Answer from the drawing. Dimensions are ordinates in mm from the lowest x, y and z of the part. A direction names the side the tool comes from. Coordinates: 2 decimals unless noted, no trailing zeros. Write each loop counter-clockwise with the first axis right and the second up, starting at its lowest first coordinate (ties: lowest second). Pieces come first, ordered by that corner, then holes. Notation, with made-up numbers: (-25, 49) - (0, 49) arc R29 cw to (0, 88) - close; hole circle Ø10 at (24.5, -8.5). An arc over 180 degrees is marked (long way). Use one line per item in the form item = value. Start each with the question number.
Item 1: A cutting plane is placed at B-B (z = 8.25). Write down the section's boundary in (x, y), then the cut area to 3 significant figures.
Item 2: Consider probe 1 along Y at (x, z) = (15, 2.75); probe 2 along Y at (x, z) = (18, 14.25); probe 3 along X at (y, z) = (169, 2). Determine where each line is inside the solid, lowest interval first.
Item 3: For the marked faces 1 and 2, determine the directions among +Z, -Z, +X, -X, +Y, -Y from which every point of the face is accessible in a straight line to the end or side of a thin tool.
Item 4: Given pin 1 (13 mm diameter, centred on x = 18, y = 19, fed in from +Z), flat-ended and moving along its own axis, determine where the tip first touches the part or whether it passes through.
Item 5: A cutting plane is placed at D-D (y = 19). Write down the section's boundary in (x, z), then the cut area to 3 significant figures.
Item 6: A cutting plane is placed at C-C (x = 18). Write down the section's boundary in (y, z), then the cut area to 3 significant figures.
Item 7: Determine the mould class of the marked faces 3, 4 and 5 for opening direction Y: released by +Y, released by -Y, zero draft, split by the parting line, or undercut.
Item 8: A cutting plane is placed at A-A (y = 163). Write down the section's boundary in (x, z), then the cut area to 3 significant figures.
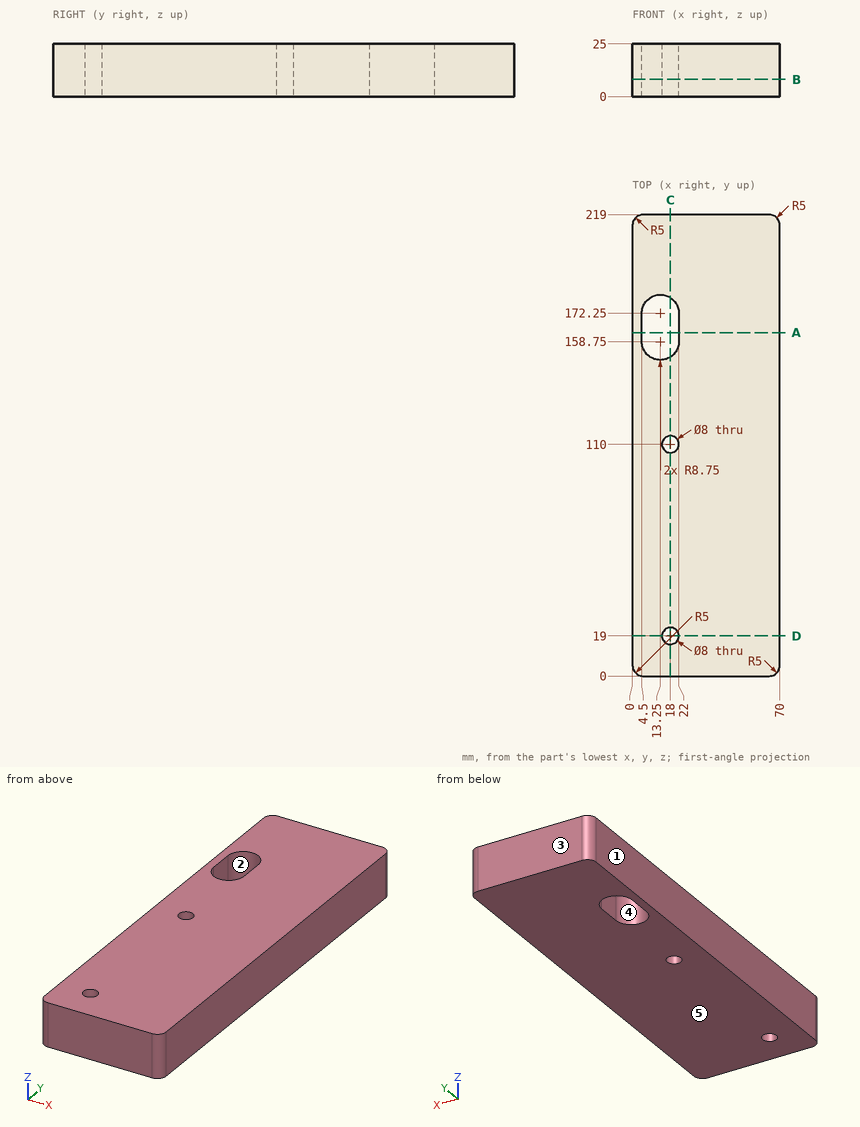
Answer:
q1.outline = (0, 5) arc R5 ccw to (5, 0) - (65, 0) arc R5 ccw to (70, 5) - (70, 214) arc R5 ccw to (65, 219) - (5, 219) arc R5 ccw to (0, 214) - close; hole (4.5, 158.75) arc R8.75 ccw to (22, 158.75) - (22, 172.25) arc R8.75 ccw to (4.5, 172.25) - close; hole circle Ø8 at (18, 19); hole circle Ø8 at (18, 110)
q1.area = 14,700 mm²
q2.probe_1 = 0 to 16.35, 21.65 to 107.35, 112.65 to 150.18, 180.82 to 219
q2.probe_2 = 0 to 15, 23 to 106, 114 to 151.4, 179.6 to 219
q2.probe_3 = 0 to 4.5, 22 to 70
q3.face_1 = +Z, -Z, -X, +Y, -Y
q3.face_2 = +Z, -Z
q4.pin_1 = 25
q5.outline = (0, 0) - (14, 0) - (14, 25) - (0, 25) - close; (22, 0) - (70, 0) - (70, 25) - (22, 25) - close
q5.area = 1,550 mm²
q6.outline = (0, 0) - (15, 0) - (15, 25) - (0, 25) - close; (23, 0) - (106, 0) - (106, 25) - (23, 25) - close; (114, 0) - (151.4, 0) - (151.4, 25) - (114, 25) - close; (179.6, 0) - (219, 0) - (219, 25) - (179.6, 25) - close
q6.area = 4,370 mm²
q7.face_3 = released by +Y
q7.face_4 = undercut
q7.face_5 = zero draft
q8.outline = (0, 0) - (4.5, 0) - (4.5, 25) - (0, 25) - close; (22, 0) - (70, 0) - (70, 25) - (22, 25) - close
q8.area = 1,310 mm²
